Could you check a few things on this model? Use its own coordinates, in mm. Round coordinates to 2 decimals unless told otherwise and drop trailing zeros. Write each loop counter-clockwise with the first axis right and the second up, starting at its lowest first coordinate (ties: lowest second). Pieces come first, ordered by that corner, then holes. Notation, with made-up numbers: (36.25, 10) - (93.25, 10) arc R26 cw to (93.25, 34) - close; hole circle Ø9 at (51, -28.75). An arc over 180 degrees is marked (long way). Write each question's results on one line, items separated by ' | '. Start each with the question number.
(1) Imagine slicing it at C-C on y = 4.5. Write out the boundary of the cut face in (x, z), then the cut area to 3 significant figures.
(2) Imagine slicing it at D-D on z = -113.5. Write out the boundary of the cut face in (x, y), then the cut area to 3 significant figures.
(3) Imagine slicing it at A-A on z = -126.5. Write out the boundary of the cut face in (x, y).
(4) Thinking about a two-plate mould opening in X: for faces 1 (the flat face through (146.188, 3, -86)), 2 (the flat face through (99, 0, -74)), 3 (the cylindrical face through (122.42, 2.96, -84.68)), which applies, +X half, -X half, draft (parallel to the pull), parting line (faces both ways), or undercut?
(5) Please list where these lines run through material, in increasing order: line 1 (X direction, y = 0.4, z = -50); line 2 (Z direction, x = 125.5, y = 4.7); line 3 (X direction, y = 1.2, z = -43). Write a range as [from, to].
(6) For P1, Ø10, axis at x = 46.19, z = -46.64, coming from the -Y side, with a flat end and sliding along its axis, tell me the tip position at first contact or that it passes through.
(7) Imagine slicing it at B-B on x = 129. Write out the boundary of the cut face in (y, z).
```python
from build123d import *

# Parameters (mm, degrees)
SKETCH_1_R      = 4.25
EXTRUDE_1_DEPTH = 6


with BuildPart() as part:
    # 草图1 → 凸台-拉伸1 (new body)
    with BuildSketch(Plane(origin=(0, 0, 0), x_dir=(1, 0, 0), z_dir=(0, 1, 0))):
        Polygon((28.188290634, 27.642710816), (146.188290634, 27.642710816), (146.188290634, 145.642710816), (106.188290634, 145.642710816), (28.188290634, 67.642710816), align=None)
        with Locations(Location((126.188290634, 126.642710816, 0), (0, 0, 270))):
            Circle(SKETCH_1_R, mode=Mode.SUBTRACT)
        with Locations(Location((126.188290634, 86.642710816, 0), (0, 0, 270))):
            Circle(SKETCH_1_R, mode=Mode.SUBTRACT)
        with Locations(Location((126.188290634, 46.642710816, 0), (0, 0, 270))):
            Circle(SKETCH_1_R, mode=Mode.SUBTRACT)
        with Locations(Location((86.188290634, 46.642710816, 0), (0, 0, 270))):
            Circle(SKETCH_1_R, mode=Mode.SUBTRACT)
        with Locations(Location((46.188290634, 46.642710816, 0), (0, 0, 270))):
            Circle(SKETCH_1_R, mode=Mode.SUBTRACT)
    extrude(amount=EXTRUDE_1_DEPTH)


solid = part.part
```
Response:
1) outline: (28.19, -67.64) - (106.19, -145.64) - (146.19, -145.64) - (146.19, -27.64) - (28.19, -27.64) - close; hole circle Ø8.5 at (46.19, -46.64); hole circle Ø8.5 at (86.19, -46.64); hole circle Ø8.5 at (126.19, -126.64); hole circle Ø8.5 at (126.19, -86.64); hole circle Ø8.5 at (126.19, -46.64) | area: 10,600 mm²
2) outline: (74.05, 0) - (146.19, 0) - (146.19, 6) - (74.05, 6) - close | area: 433 mm²
3) outline: (87.05, 0) - (121.94, 0) - (121.94, 6) - (87.05, 6) - close; (130.44, 0) - (146.19, 0) - (146.19, 6) - (130.44, 6) - close
4) face 1: +X half | face 2: draft | face 3: undercut
5) line 1: [28.19, 43.58], [48.79, 83.58], [88.79, 123.58], [128.79, 146.19] | line 2: [-145.64, -130.84], [-122.45, -90.84], [-82.45, -50.84], [-42.45, -27.64] | line 3: [28.19, 44], [48.38, 84], [88.38, 124], [128.38, 146.19]
6) P1: y = 0
7) outline: (0, -145.64) - (6, -145.64) - (6, -129.83) - (0, -129.83) - close; (0, -123.46) - (6, -123.46) - (6, -89.83) - (0, -89.83) - close; (0, -83.46) - (6, -83.46) - (6, -49.83) - (0, -49.83) - close; (0, -43.46) - (6, -43.46) - (6, -27.64) - (0, -27.64) - close
